Design review of the part built by this model. Coordinates are the model's own, in mm. Round coordinates to 2 decimals unless told otherwise and drop trailing zeros. Order: outer loops, then holes, each group sorted by start corner. A loop starts at its lowest first (then second) coordinate and runs counter-clockwise, first axis right, second up. Notation, with made-up numbers: (60.25, 48.5) - (80.25, 48.5) arc R12 cw to (80.25, 55.5) - close; hole circle Ø7 at (81.5, -20). An arc over 180 degrees is marked (long way). Answer as a JSON object with one key per item and string values. Group by question number.
from build123d import *

# Parameters (mm, degrees)
SKETCH1_R           = 11.1125
BOSS_EXTRUDE1_DEPTH = 5.55625
SKETCH2_R           = 7
CUT_EXTRUDE1_DEPTH  = 5.55625
FILLET1_R           = 10
SKETCH3_R           = 2.25
SKETCH3_R_2         = 2
CUT_EXTRUDE2_DEPTH  = 6.35
SKETCH4_R           = 2.5
CUT_EXTRUDE3_DEPTH  = 40


with BuildPart() as part:
    # Sketch1 → Boss-Extrude1 (new body)
    with BuildSketch(Plane.XY):
        with BuildLine():
            Line((-65, 47), (94.62424518, 47))
            Line((94.62424518, 47), (94.62424518, -47))
            Line((94.62424518, -47), (-65, -47))
            ThreePointArc((-65, -47), (-112, 0), (-65, 47))
        make_face()
        with Locations((-65, 0)):
            Circle(SKETCH1_R, mode=Mode.SUBTRACT)
    extrude(amount=BOSS_EXTRUDE1_DEPTH)

    # Sketch2 → Cut-Extrude1 (cut)
    with BuildSketch(Plane.XY.offset(5.55625)):
        with Locations((33.666397681, 0)):
            Circle(SKETCH2_R)
    extrude(amount=-CUT_EXTRUDE1_DEPTH, mode=Mode.SUBTRACT)

    # Fillet1
    fillet1_edges = [part.edges().sort_by_distance(p)[0] for p in [
        (94.62424518, 47, 2.778125),
        (94.62424518, -47, 2.778125),
    ]]
    fillet(fillet1_edges, radius=FILLET1_R)

    # Sketch3 → Cut-Extrude2 (cut)
    with BuildSketch(Plane.XY.offset(5.55625)):
        with Locations((78.666397681, 30)):
            Circle(SKETCH3_R)
        with Locations((78.666397681, -30)):
            Circle(SKETCH3_R)
        with Locations((-11.333602319, 30)):
            Circle(SKETCH3_R)
        with Locations((-11.333602319, -30)):
            Circle(SKETCH3_R)
        with Locations((-11.333602319, 41)):
            Circle(SKETCH3_R_2)
        with Locations((-11.333602319, -41)):
            Circle(SKETCH3_R_2)
    extrude(amount=-CUT_EXTRUDE2_DEPTH, mode=Mode.SUBTRACT)

    # Sketch4 → Cut-Extrude3 (cut)
    with BuildSketch(Plane.XY.offset(5.55625)):
        with Locations((0, 17.5)):
            Circle(SKETCH4_R)
        with Locations((0, -17.5)):
            Circle(SKETCH4_R)
    extrude(amount=-CUT_EXTRUDE3_DEPTH, mode=Mode.SUBTRACT)


solid = part.part
1. Clearance check with flat-ended pins moving along their axes: P1, Ø4.5, axis at x = -11.33, y = 41, coming from the +Z side; P2, Ø4, axis at x = -11.33, y = 30, coming from the +Z side; P3, Ø1.5, axis at y = 23, z = 1.5, coming from the -X side. State where each tip first meets the part, or that it passes through.
2. To check wall thickness, follow line 1 (Y direction, x = -10, z = 3.2); line 2 (Y direction, x = 0, z = 1.95); line 3 (X direction, y = 9, z = 3.8). State the ranges of each line that lie inside material, in increasing order. Write a range as from..to.
3. Mouldability with a two-part tool opening along X and no side actions: class faces 1 (the cylindrical face through (91.617, 44.148, 2.817)), 2 (the flat face through (-7, 1, 0)), 3 (the cylindrical face through (-76.1, 0.5, 2.7)) as pulls with the +X half, pulls with the -X half, needs draft (parallel to the pull), parting line crosses it, or undercut.
4. Take a section at D-D, the plane x = 34.5. Give the boundary of the cut face in (y, z), then the cut area to 3 significant figures.
5. Take a section at C-C, the plane y = 4. Give the boundary of the cut face in (x, z).
6. Take a section at B-B, the plane z = 4.3. Count the separate pieces of the cut face and the enclosed holes in it, then the cut area to 3 significant figures.
7. Take a section at A-A, the plane x = 0. Give the boundary of the cut face in (y, z), then the cut area to 3 significant figures.
Response values:
{
 "1": {"P1": "z = 5.56", "P2": "through", "P3": "x = -106.4"},
 "2": {"line 1": "-47..-42.49, -39.51..-31.81, -28.19..28.19, 31.81..39.51, 42.49..47", "line 2": "-47..-20, -15..15, 20..47", "line 3": "-111.13..-71.52, -58.48..94.62"},
 "3": {"face 1": "pulls with the +X half", "face 2": "needs draft", "face 3": "undercut"},
 "4": {"outline": "(-47, 0) - (-6.95, 0) - (-6.95, 5.56) - (-47, 5.56) - close; (6.95, 0) - (47, 0) - (47, 5.56) - (6.95, 5.56) - close", "area": "445 mm2"},
 "5": {"outline": "(-111.83, 0) - (-75.37, 0) - (-75.37, 5.56) - (-111.83, 5.56) - close; (-54.63, 0) - (27.92, 0) - (27.92, 5.56) - (-54.63, 5.56) - close; (39.41, 0) - (94.62, 0) - (94.62, 5.56) - (39.41, 5.56) - close"},
 "6": {"separate pieces": "1", "enclosed holes": "10", "area": "17,800 mm2"},
 "7": {"outline": "(-47, 0) - (-20, 0) - (-20, 5.56) - (-47, 5.56) - close; (-15, 0) - (15, 0) - (15, 5.56) - (-15, 5.56) - close; (20, 0) - (47, 0) - (47, 5.56) - (20, 5.56) - close", "area": "467 mm2"}
}
